Input: part model. Units: mm. Frame: model coordinates. Face numbers are marked on the shaded views. A direction names the side the tool comes from. Round coordinates to 2 decimals unless told otherwise and drop trailing zeros. Order: outer loops, then holes, each group sorted by start corner. A loop starts at its lowest first (then second) coordinate and runs counter-clockwise, first axis right, second up. Notation, with made-up numbers: (34, 81) -> (57, 81) arc R16 cw to (57, 98) -> close; hole circle Ø8 at (59, -31). An arc over 180 degrees is marked (long way). Answer as CSV lines item,"result". Start each with the question number.
1) Mould query, pull axis X, two halves, no side actions, for the marked faces 1, 2 and 3. Classes: +X half, -X half, draft (parallel to the pull), parting line (faces both ways), or undercut.
2) Line query: L1, parallel to Y at x = 0, z = 19.95 (3 decimals); L2, parallel to Y at x = 2, z = 14.75; L3, parallel to X at y = 0, z = 1.85. Output: solid intervals per line, ascending.
3) Section query B-B, the plane y = 7. Output: boundary loops of the cut face in (x, z), and give its area (3 significant figures).
4) Section query C-C, the plane x = -20. Output: boundary loops of the cut face in (y, z), and give its area (3 significant figures).
5) First-contact query: P1, Ø8.5, axis at x = 9, z = 9, coming from the +Y side; P2, Ø2, axis at y = -12.5, z = 3, coming from the -X side; P3, Ø1.2, axis at x = -7, y = -2.5, coming from the -Z side; P4, Ø3, axis at x = 0, y = -0.475, coming from the +Z side. Flat tips, straight axial feed; report the tip coordinate or a pass-through.
6) Section query A-A, the plane z = 18. State how many separate pieces and enclosed holes the cut face has, and give its area (3 significant figures).
7) Access query for the marked faces 4, 5, 6 and 7. Directions: +Z, -Z, +X, -X, +Y, -Y. A direction counts if a zero-diameter tool reaches every point of the face in a straight line with its end or side. Return the directions, or none.
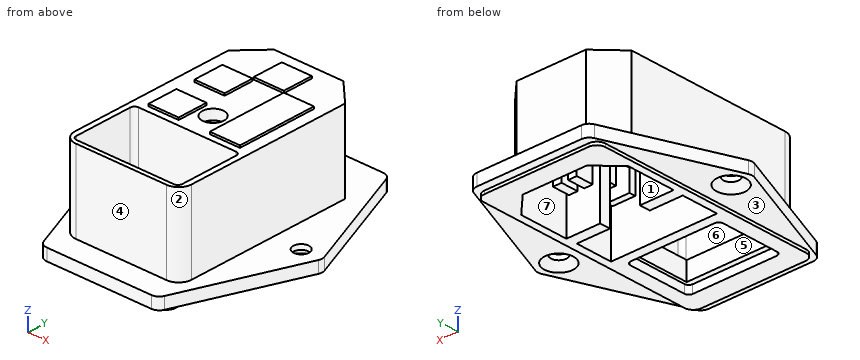
```python
from build123d import *

# Parameters (mm, degrees)
SKETCH1_W                    = 27
SKETCH1_H                    = 58
BOSS_EXTRUDE1_DEPTH          = 2.7
FILLET1_R                    = 2
BOSS_EXTRUDE2_DEPTH          = 0.7
SKETCH5_W                    = 27.1
SKETCH5_H                    = 46.9
BOSS_EXTRUDE3_DEPTH          = 18.6
FILLET2_R                    = 3
CHAMFER1_SIZE                = 5.5
CUT_EXTRUDE1_DEPTH           = 15.8
SKETCH7_W                    = 9.25
SKETCH7_H                    = 2.45
SKETCH7_W_2                  = 24.6
SKETCH7_H_2                  = 8.55
CUT_EXTRUDE2_DEPTH           = 19.7
SKETCH8_R                    = 2.5
CUT_EXTRUDE3_DEPTH           = 43.971353827
SKETCH9_W                    = 20
SKETCH9_H                    = 13
CUT_EXTRUDE4_DEPTH           = 45.073203307
CUT_EXTRUDE5_DEPTH           = 1.9
SKETCH11_W                   = 7
SKETCH11_H                   = 7
SKETCH11_H_2                 = 18.5
BOSS_EXTRUDE4_DEPTH          = 0.5
SKETCH12_W                   = 5.3
SKETCH12_H                   = 1.45
BOSS_EXTRUDE5_DEPTH          = 9.9
SKETCH12_3_W                 = 2
SKETCH12_3_H                 = 4
BOSS_EXTRUDE6_DEPTH          = 14.6
SKETCH12_4_W                 = 2
SKETCH12_4_H                 = 4
BOSS_EXTRUDE7_DEPTH          = 17.5
CSK_FOR_M3_SFHCS1_AT_2_COUNT = 2
CSK_FOR_M3_SFHCS1_AT_2_PITCH = 40


with BuildPart() as part:
    # Sketch1 → Boss-Extrude1 (new body)
    with BuildSketch(Plane.XY):
        Polygon((-13.5, 29), (-25, 0), (-13.5, -29), align=None)
        Rectangle(SKETCH1_W, SKETCH1_H)
        Polygon((13.5, 29), (25, 0), (13.5, -29), align=None)
    extrude(amount=BOSS_EXTRUDE1_DEPTH)

    # Fillet1
    fillet1_edges = [part.edges().sort_by_distance(p)[0] for p in [
        (-13.5, 29, 1.35),
        (13.5, 29, 1.35),
        (25, 0, 1.35),
        (13.5, -29, 1.35),
        (-13.5, -29, 1.35),
        (-25, 0, 1.35),
    ]]
    fillet(fillet1_edges, radius=FILLET1_R)

    # Sketch2 → Boss-Extrude2 (add)
    with BuildSketch(Plane(origin=(0, 0, 0), x_dir=(-1, 0, 0), z_dir=(0, 0, -1))):
        with BuildLine():
            Line((-12.1, -27.1), (12.1, -27.1))
            ThreePointArc((12.1, -27.1), (13.514213562, -26.514213562), (14.1, -25.1))
            Line((14.1, -25.1), (14.1, 25.1))
            ThreePointArc((14.1, 25.1), (13.514213562, 26.514213562), (12.1, 27.1))
            Line((12.1, 27.1), (-12.1, 27.1))
            ThreePointArc((-12.1, 27.1), (-13.514213562, 26.514213562), (-14.1, 25.1))
            Line((-14.1, 25.1), (-14.1, -25.1))
            ThreePointArc((-14.1, -25.1), (-13.514213562, -26.514213562), (-12.1, -27.1))
        make_face()
    extrude(amount=BOSS_EXTRUDE2_DEPTH)

    # Sketch5 → Boss-Extrude3 (add)
    with BuildSketch(Plane.XY.offset(2.7)):
        Rectangle(SKETCH5_W, SKETCH5_H)
    extrude(amount=BOSS_EXTRUDE3_DEPTH)

    # Fillet2
    fillet2_edges = [part.edges().sort_by_distance(p)[0] for p in [
        (13.55, -23.45, 12),
        (-13.55, -23.45, 12),
    ]]
    fillet(fillet2_edges, radius=FILLET2_R)

    # Chamfer1
    chamfer1_edges = [part.edges().sort_by_distance(p)[0] for p in [
        (13.55, 23.45, 12),
        (-13.55, 23.45, 12),
    ]]
    chamfer(chamfer1_edges, length=CHAMFER1_SIZE)

    # Sketch6 → Cut-Extrude1 (cut)
    with BuildSketch(Plane.XY.offset(21.3)):
        with BuildLine():
            Line((-11.3, -22.45), (11.3, -22.45))
            ThreePointArc((11.3, -22.45), (12.007106781, -22.157106781), (12.3, -21.45))
            Line((12.3, -21.45), (12.3, -7.95))
            ThreePointArc((12.3, -7.95), (12.007106781, -7.242893219), (11.3, -6.95))
            Line((11.3, -6.95), (-11.3, -6.95))
            ThreePointArc((-11.3, -6.95), (-12.007106781, -7.242893219), (-12.3, -7.95))
            Line((-12.3, -7.95), (-12.3, -21.45))
            ThreePointArc((-12.3, -21.45), (-12.007106781, -22.157106781), (-11.3, -22.45))
        make_face()
    extrude(amount=-CUT_EXTRUDE1_DEPTH, mode=Mode.SUBTRACT)

    # Sketch7 → Cut-Extrude2 (cut)
    with BuildSketch(Plane(origin=(0, 0, -0.7), x_dir=(-1, 0, 0), z_dir=(0, 0, -1))):
        Polygon((-12.45, 6.25), (12.45, 6.25), (12.45, 17.55), (7.45, 22.55), (-7.45, 22.55), (-12.45, 17.55), align=None)
        with Locations((0, 5.025)):
            Rectangle(SKETCH7_W, SKETCH7_H)
        with Locations((0, -0.475)):
            Rectangle(SKETCH7_W_2, SKETCH7_H_2)
    extrude(amount=-CUT_EXTRUDE2_DEPTH, mode=Mode.SUBTRACT)

    # Sketch8 → Cut-Extrude3 (cut, through all)
    with BuildSketch(Plane(origin=(0, 0, 19), x_dir=(-1, 0, 0), z_dir=(0, 0, -1))):
        with Locations((0, -0.475)):
            Circle(SKETCH8_R)
    extrude(amount=-CUT_EXTRUDE3_DEPTH, mode=Mode.SUBTRACT)

    # Sketch9 → Cut-Extrude4 (cut, through all)
    with BuildSketch(Plane(origin=(0, 0, -0.7), x_dir=(-1, 0, 0), z_dir=(0, 0, -1))):
        with Locations((0, -14.7)):
            Rectangle(SKETCH9_W, SKETCH9_H)
    extrude(amount=-CUT_EXTRUDE4_DEPTH, mode=Mode.SUBTRACT)

    # Sketch10 → Cut-Extrude5 (cut)
    with BuildSketch(Plane(origin=(0, 0, -0.7), x_dir=(-1, 0, 0), z_dir=(0, 0, -1))):
        with BuildLine():
            Line((-9.75, -22.45), (9.75, -22.45))
            ThreePointArc((9.75, -22.45), (10.457106781, -22.157106781), (10.75, -21.45))
            Line((10.75, -21.45), (10.75, -7.95))
            ThreePointArc((10.75, -7.95), (10.457106781, -7.242893219), (9.75, -6.95))
            Line((9.75, -6.95), (-9.75, -6.95))
            ThreePointArc((-9.75, -6.95), (-10.457106781, -7.242893219), (-10.75, -7.95))
            Line((-10.75, -7.95), (-10.75, -21.45))
            ThreePointArc((-10.75, -21.45), (-10.457106781, -22.157106781), (-9.75, -22.45))
        make_face()
    extrude(amount=-CUT_EXTRUDE5_DEPTH, mode=Mode.SUBTRACT)

    # Sketch11 → Boss-Extrude4 (add)
    with BuildSketch(Plane.XY.offset(21.3)):
        with Locations((0, 16.95)):
            Rectangle(SKETCH11_W, SKETCH11_H)
        with Locations((7.45, 3.7)):
            Rectangle(SKETCH11_W, SKETCH11_H_2)
        with Locations((-6.8, 9.45)):
            Rectangle(SKETCH11_W, SKETCH11_H)
        with Locations((-6.8, -2.05)):
            Rectangle(SKETCH11_W, SKETCH11_H)
    extrude(amount=BOSS_EXTRUDE4_DEPTH)

    # Sketch12 → Boss-Extrude5 (add)
    with BuildSketch(Plane(origin=(0, 0, 19), x_dir=(-1, 0, 0), z_dir=(0, 0, -1))):
        with Locations((-8.25, 1.95)):
            Rectangle(SKETCH12_W, SKETCH12_H)
        with Locations((-8.25, -2.9)):
            Rectangle(SKETCH12_W, SKETCH12_H)
        with Locations((8.25, 1.95)):
            Rectangle(SKETCH12_W, SKETCH12_H)
        with Locations((8.25, -2.9)):
            Rectangle(SKETCH12_W, SKETCH12_H)
    extrude(amount=BOSS_EXTRUDE5_DEPTH)

    # Sketch12<3> → Boss-Extrude6 (add)
    with BuildSketch(Plane(origin=(0, 0, 19), x_dir=(-1, 0, 0), z_dir=(0, 0, -1))):
        with Locations((-7, 12.4)):
            Rectangle(SKETCH12_3_W, SKETCH12_3_H)
        with Locations((7, 12.4)):
            Rectangle(SKETCH12_3_W, SKETCH12_3_H)
    extrude(amount=BOSS_EXTRUDE6_DEPTH)

    # Sketch12<4> → Boss-Extrude7 (add)
    with BuildSketch(Plane(origin=(0, 0, 19), x_dir=(-1, 0, 0), z_dir=(0, 0, -1))):
        with Locations((0, 16.15)):
            Rectangle(SKETCH12_4_W, SKETCH12_4_H)
    extrude(amount=BOSS_EXTRUDE7_DEPTH)

    # Sketch16 → CSK for M3 SFHCS1 (revolve, cut)
    with BuildSketch(Plane.YZ.offset(20)):
        Polygon((0, 0), (0, 2.7), (1.8, 2.7), (1.8, 1.56), (3.36, 0), align=None)
    csk_for_m3_sfhcs1 = revolve(axis=Axis((20, 0, -6.35), (0, 0, 1)), mode=Mode.SUBTRACT)

    # CSK for M3 SFHCS1 at 2: CSK for M3 SFHCS1 ×2
    with Locations(*[(-i * CSK_FOR_M3_SFHCS1_AT_2_PITCH, 0, 0) for i in range(1, CSK_FOR_M3_SFHCS1_AT_2_COUNT)]):
        add(csk_for_m3_sfhcs1, mode=Mode.SUBTRACT)


solid = part.part
```
Findings:
1,face 1,"undercut"
1,face 2,"+X half"
1,face 3,"draft"
2,L1,"y = -23.45 to -22.45, -6.95 to -2.975, 2.025 to 23.45"
2,L2,"y = -23.45 to -22.45, -6.95 to -4.75, 22.55 to 23.45"
2,L3,"x = -24.85 to -21.8, -18.2 to -12.3, 12.3 to 18.2, 21.8 to 24.85"
3,outline,"(-22.22, 0) -> (-14.1, 0) -> (-14.1, -0.7) -> (-12.45, -0.7) -> (-12.45, 19) -> (12.45, 19) -> (12.45, -0.7) -> (14.1, -0.7) -> (14.1, 0) -> (22.22, 0) -> (22.22, 2.7) -> (13.55, 2.7) -> (13.55, 21.3) -> (10.95, 21.3) -> (10.95, 21.8) -> (3.95, 21.8) -> (3.95, 21.3) -> (-3.3, 21.3) -> (-3.3, 21.8) -> (-10.3, 21.8) -> (-10.3, 21.3) -> (-13.55, 21.3) -> (-13.55, 2.7) -> (-22.22, 2.7) -> close"
3,area,"160 mm^2"
4,outline,"(-12.61, 0) -> (-3.36, 0) -> (-1.8, 1.56) -> (-1.8, 2.7) -> (-12.61, 2.7) -> close; (1.8, 1.56) -> (3.36, 0) -> (12.61, 0) -> (12.61, 2.7) -> (1.8, 2.7) -> close"
4,area,"55.9 mm^2"
5,P1,"stops at y = 23.45"
5,P2,"stops at x = -20.42"
5,P3,"stops at z = 9.1"
5,P4,"passes through"
6,separate pieces,"8"
6,enclosed holes,"2"
6,area,"297 mm^2"
7,face 4,"+Z, +X, -X, -Y"
7,face 5,"+Z, -Z"
7,face 6,"+Z"
7,face 7,"-Z"
